Work out the finished part from the listing and answer in its coordinate system (mm). A direction names the side the tool comes from. Give positions to 0.01 mm unless a question says otherwise; leave off trailing zeros. Write each loop counter-clockwise with the first axis right and the second up, starting at its lowest first coordinate (ties: lowest second). Pieces come first, ordered by that corner, then holes.
1) Find section B-B (y = 17.25). Determine the outline of the cut face in (x, z), plus the area to 3 significant figures.
2) Find section A-A (z = 0). Determine the outline of the cut face in (x, y), plus the area to 3 significant figures.
3) Straight lines are drawn through the part: probe 1 along Y at (x, z) = (0, -59.1); probe 2 along X at (y, z) = (11.5, 0); probe 3 along Z at (x, y) = (6, 1.5). For each, find the intervals that lie inside material, in ascending order.
4) A tool of negligible diameter and unlimited length cuts with its end or side. For faces 4 (the face through (5, 6, -55)), 5 (the face through (24.09, 23.96, -26.28)), 6 (the face through (4, 15, -55)), from which of +Z, -Z, +X, -X, +Y, -Y can it reach the whole face along a straight path? Write none if from no direction.
5) Given pin 1 Ø2 at (y, z) = (10, -53.5) entering from -X; pin 2 Ø2 at (x, z) = (-0.5, -58.5) entering from +Y; pin 3 Ø6 at (x, y) = (0, 10) entering from -Z, each flat-ended and moving along its own axis, determine where each tip first touches the part or whether it passes through.
6) Determine the mould class of faces 1 (the face through (24, 21.5, -27)), 2 (the face through (0.488, 13.718, -60.042)), 3 (the face through (-3.26, 3.5, -45.04)) for opening direction Y: pulls with the +Y half, pulls with the -Y half, needs draft (parallel to the pull), parting line crosses it, or undercut.
```python
from build123d import *

# Parameters (mm, degrees)
SKETCH_1_R           = 47
EXTRUDE_1_DEPTH      = 21.5
SKETCH_2_R           = 35.65
EXTRUDE_2_DEPTH      = 7
SKETCH_3_R           = 30.25
CUT_EXTRUDE_1_DEPTH  = 73.320467366
FILLET_1_R           = 2
EXTRUDE_3_DEPTH      = 6
EXTRUDE_3_DEPTH_BACK = 6
SKETCH_4_W           = 103.611126825
SKETCH_4_H           = 12
CUT_EXTRUDE_3_DEPTH  = 81.212218579
FILLET_2_R           = 5
SKETCH_5_R           = 3.75
CUT_EXTRUDE_2_DEPTH  = 6
SKETCH_7_R           = 47
SKETCH_7_R_2         = 45
CUT_EXTRUDE_4_DEPTH  = 3.5
FILLET_3_R           = 3


with BuildPart() as part:
    # Sketch 1 → Extrude 1 (new body)
    with BuildSketch(Plane(origin=(0, 0, 0), x_dir=(1, 0, 0), z_dir=(0, 1, 0))):
        with Locations(Location((0, 0, 0), (0, 0, 270))):
            Circle(SKETCH_1_R)
    extrude(amount=EXTRUDE_1_DEPTH)

    # Sketch 2 → Extrude 2 (add)
    with BuildSketch(Plane(origin=(0, 21.5, 0), x_dir=(1, 0, 0), z_dir=(0, 1, 0))):
        with Locations(Location((0, 0, 0), (0, 0, 270))):
            Circle(SKETCH_2_R)
    extrude(amount=EXTRUDE_2_DEPTH)

    # Sketch 3 → Cut-Extrude 1 (cut, through all)
    with BuildSketch(Plane(origin=(0, 28.5, 0), x_dir=(1, 0, 0), z_dir=(0, 1, 0))):
        with Locations(Location((0, 0, 0), (0, 0, 270))):
            Circle(SKETCH_3_R)
    extrude(amount=-CUT_EXTRUDE_1_DEPTH, mode=Mode.SUBTRACT)

    # Fillet 1
    fillet_1_edges = [part.edges().sort_by_distance(p)[0] for p in [
        (0, 21.5, -47),
        (0, 28.5, -35.65),
    ]]
    fillet(fillet_1_edges, radius=FILLET_1_R)

    # Sketch 4 → Extrude 3 (add, two sides: drawn at the far end of the back side and taken through both)
    with BuildSketch(Plane(origin=(0, 0, 0), x_dir=(0, 0, -1), z_dir=(1, 0, 0)).offset(-EXTRUDE_3_DEPTH_BACK)):
        with Locations((11.194436588, 10)):
            Rectangle(SKETCH_4_W, SKETCH_4_H)
    extrude(amount=EXTRUDE_3_DEPTH + EXTRUDE_3_DEPTH_BACK)

    # Sketch 6 → Cut-Extrude 3 (cut, through all)
    with BuildSketch(Plane(origin=(0, 16, 0), x_dir=(1, 0, 0), z_dir=(0, 1, 0))):
        with BuildLine():
            Line((-6, 29.648988178), (-6, -29.648988178))
            ThreePointArc((-6, -29.648988178), (0, -30.25), (6, -29.648988178))
            Line((6, -29.648988178), (6, 29.648988178))
            ThreePointArc((6, 29.648988178), (0, 30.25), (-6, 29.648988178))
        make_face()
    extrude(amount=-CUT_EXTRUDE_3_DEPTH, mode=Mode.SUBTRACT)

    # Fillet 2
    fillet_2_edges = [part.edges().sort_by_distance(p)[0] for p in [
        (-6, 16, -54.807724042),
        (-6, 4, -54.807724042),
        (6, 4, -54.807724042),
        (6, 16, -54.807724042),
    ]]
    fillet(fillet_2_edges, radius=FILLET_2_R)

    # Sketch 5 → Cut-Extrude 2 (cut)
    with BuildSketch(Plane(origin=(0, 0, -63), x_dir=(-1, 0, 0), z_dir=(0, 0, -1))):
        with Locations((0, 10)):
            Circle(SKETCH_5_R)
    extrude(amount=-CUT_EXTRUDE_2_DEPTH, mode=Mode.SUBTRACT)

    # Sketch 7 → Cut-Extrude 4 (cut)
    with BuildSketch(Plane.XZ):
        with Locations(Location((0, 0, 0), (0, 0, 270))):
            Circle(SKETCH_7_R)
        with Locations(Location((0, 0, 0), (0, 0, 270))):
            Circle(SKETCH_7_R_2, mode=Mode.SUBTRACT)
    extrude(amount=-CUT_EXTRUDE_4_DEPTH, mode=Mode.SUBTRACT)

    # Fillet 3
    fillet_3_edges = [part.edges().sort_by_distance(p)[0] for p in [
        (0, 0, 45),
    ]]
    fillet(fillet_3_edges, radius=FILLET_3_R)


solid = part.part
```
Results:
1. outline: circle Ø94 at (0, 0); hole circle Ø60.5 at (0, 0)
1. area: 4,070 mm2
2. outline: (-47, 3.5) - (-45, 3.5) - (-45, 3) arc R3 ccw to (-42, 0) - (-30.25, 0) - (-30.25, 28.5) - (-33.65, 28.5) arc R2 ccw to (-35.65, 26.5) - (-35.65, 21.5) - (-45, 21.5) arc R2 ccw to (-47, 19.5) - close; (30.25, 0) - (42, 0) arc R3 ccw to (45, 3) - (45, 3.5) - (47, 3.5) - (47, 19.5) arc R2 ccw to (45, 21.5) - (35.65, 21.5) - (35.65, 26.5) arc R2 ccw to (33.65, 28.5) - (30.25, 28.5) - close
2. area: 775 mm2
3. probe 1: y = 4 to 6.25, 13.75 to 16
3. probe 2: x = -47 to -30.25, 30.25 to 47
3. probe 3: z = -44.19 to -29.65, 29.65 to 44.19
4. face 4: -Z, +X, -Y
4. face 5: +Y
4. face 6: -Z, +X, +Y
5. pin 1: stops at x = -6
5. pin 2: stops at y = 16
5. pin 3: stops at z = -57
6. face 1: pulls with the +Y half
6. face 2: undercut
6. face 3: pulls with the -Y half
